Source: CAD feature listing. Evaluate the final solid. Frame: model axes, mm. Face numbers are marked on the shaded views. A direction names the side the tool comes from. Round coordinates to 2 decimals unless told otherwise and drop trailing zeros. Write each loop counter-clockwise with the first axis right and the second up, starting at its lowest first coordinate (ties: lowest second). Pieces come first, ordered by that corner, then holes. Notation, with made-up numbers: M -0.5,65 L 26.5,65 A32 cw 26.5,99 Z; hole C -18,80.25 d9. An arc over 180 degrees is marked long. Put each result on its own line as item: value. Start each with the question number.
```python
from build123d import *

# Parameters (mm, degrees)
SKETCH1_W                 = 23.7998
SKETCH1_H                 = 9.525
BOSS_EXTRUDE1_DEPTH       = 12.192
SKETCH2_W                 = 11.0998
SKETCH2_H                 = 9.525
CUT_EXTRUDE1_DEPTH        = 5.842
FILLET1_R                 = 1.5748
F_4_40_TAPPED_HOLE5_D     = 2.2606
F_4_40_TAPPED_HOLE5_DEPTH = 6.35
F_4_40_TAPPED_HOLE5_TIP   = 0.679152758
SKETCH4_R                 = 1.5875
SKETCH4_R_2               = 1.143
CUT_EXTRUDE2_DEPTH        = 18.689937543
F_10_32_TAPPED_HOLE1_D    = 4.0386


with BuildPart() as part:
    # Sketch1 → Boss-Extrude1 (new body)
    with BuildSketch(Plane(origin=(0, 0, 0), x_dir=(1, 0, 0), z_dir=(0, 1, 0))):
        Rectangle(SKETCH1_W, SKETCH1_H)
    extrude(amount=BOSS_EXTRUDE1_DEPTH)

    # Sketch2 → Cut-Extrude1 (cut)
    with BuildSketch(Plane(origin=(0, 12.192, 0), x_dir=(1, 0, 0), z_dir=(0, 1, 0))):
        with Locations((6.35, 0)):
            Rectangle(SKETCH2_W, SKETCH2_H)
    extrude(amount=-CUT_EXTRUDE1_DEPTH, mode=Mode.SUBTRACT)

    # Fillet1
    fillet1_edges = [part.edges().sort_by_distance(p)[0] for p in [
        (0.8001, 6.35, 0),
    ]]
    fillet(fillet1_edges, radius=FILLET1_R)

    # #4-40 Tapped Hole5
    with Locations(Plane(origin=(-2.3749, 12.192, 0), x_dir=(0, 0, 1), z_dir=(0, 1, 0))):
        with Locations((0, 0)):
            Hole(F_4_40_TAPPED_HOLE5_D / 2, depth=F_4_40_TAPPED_HOLE5_DEPTH)
            with Locations((0, 0, -(F_4_40_TAPPED_HOLE5_DEPTH + F_4_40_TAPPED_HOLE5_TIP / 2))):  # 118° drill point
                Cone(0, F_4_40_TAPPED_HOLE5_D / 2, F_4_40_TAPPED_HOLE5_TIP, mode=Mode.SUBTRACT)

    # Sketch4 → Cut-Extrude2 (cut, through all)
    with BuildSketch(Plane(origin=(0, 12.192, 0), x_dir=(1, 0, 0), z_dir=(0, 1, 0))):
        with Locations(Location((-8.7249, 0, 0), (0, 0, 270))):
            Circle(SKETCH4_R)
        with Locations(Location((-2.3749, 0, 0), (0, 0, 270))):
            Circle(SKETCH4_R_2)
    extrude(amount=-CUT_EXTRUDE2_DEPTH, mode=Mode.SUBTRACT)

    # #10-32 Tapped Hole1 (through all)
    with Locations(Plane(origin=(0, 6.35, 0), x_dir=(1, 0, 0), z_dir=(0, 1, 0))):
        with Locations((7.1374, 0)):
            Hole(F_10_32_TAPPED_HOLE1_D / 2)


solid = part.part
```
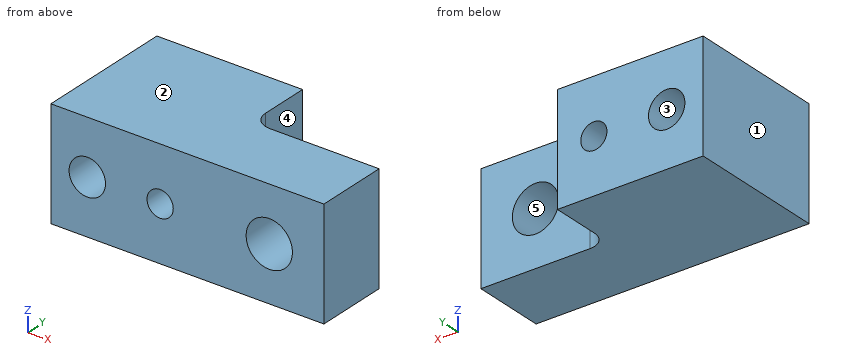
(1) Section query C-C (z = 3.75). Return loops of the section in (x, y).
(2) Access query for the marked faces 4 and 5. Directions: +Z, -Z, +X, -X, +Y, -Y. A direction counts if a zero-diameter tool reaches every point of the face in a straight line with its end or side. Return the directions, or none.
(3) Section query B-B (x = 7). Return loops of the section in (y, z), and give its area (3 significant figures).
(4) Pull-direction query (X, two-part tool) for the marked faces 1, 2 and 3; classes: +X half, -X half, draft (parallel to the pull), parting line (faces both ways), or undercut.
(5) Section query A-A (z = 0). Return loops of the section in (x, y), and give its area (3 significant figures).
(6) Ray query, line 1 along X through (y, z) = (8, 0); line 2 along X through (y, z) = (6.75, -0.5); line 3 along Y through (x, z) = (2.5, -0.5). Return the intervals inside material, ascending.
(7) Section query D-D (y = 5.5). Return loops of the section in (x, z) (1 decimal), and give its area (3 significant figures).
(8) Contact query for flat-ended pins moving along their axis: P1, Ø1.8, axis at x = -2.37, z = 0, coming from the -Y side; P2, Ø4.5, axis at y = 11, z = 1, coming from the +X side. Output: stop coordinate, or through.
Entries:
1. outline: M -11.9,0 L 11.9,0 L 11.9,6.35 L 2.37,6.35 A1.57 cw 0.8,7.92 L 0.8,12.19 L -11.9,12.19 Z
2. face 4: +Z, -Z, +X, +Y
2. face 5: +Y, -Y
3. outline: M 0,-4.76 L 6.35,-4.76 L 6.35,-2.01 L 0,-2.01 Z; M 0,2.01 L 6.35,2.01 L 6.35,4.76 L 0,4.76 Z
3. area: 34.9 mm2
4. face 1: -X half
4. face 2: draft
4. face 3: undercut
5. outline: M -11.9,0 L -10.31,0 L -10.31,12.19 L -11.9,12.19 Z; M -7.14,0 L -3.52,0 L -3.52,12.19 L -7.14,12.19 Z; M -1.23,0 L 5.12,0 L 5.12,6.35 L 2.37,6.35 A1.57 cw 0.8,7.92 L 0.8,12.19 L -1.23,12.19 Z; M 9.16,0 L 11.9,0 L 11.9,6.35 L 9.16,6.35 Z
5. area: 134 mm2
6. line 1: -11.9 to -10.31, -7.14 to -3.52, -1.23 to 0.8
6. line 2: -11.9 to -10.23, -7.22 to -3.4, -1.35 to 1.33
6. line 3: 0 to 6.35
7. outline: M -11.9,-4.8 L 11.9,-4.8 L 11.9,4.8 L -11.9,4.8 Z; hole C -8.7,0 d3.2; hole C -2.4,0 d2.3; hole C 7.1,0 d4
7. area: 202 mm2
8. P1: through
8. P2: x = 0.8
